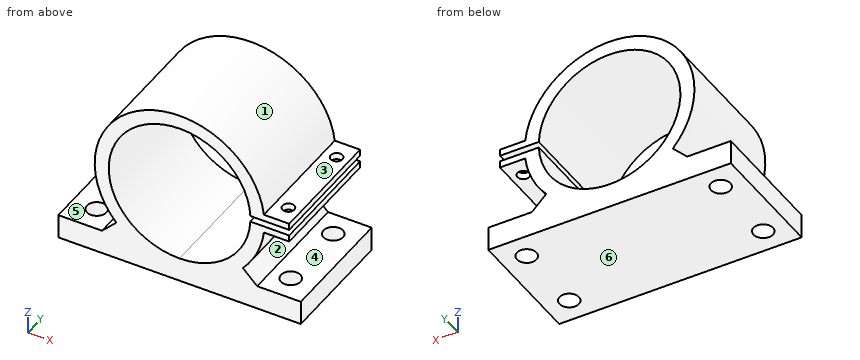
from build123d import *

# Parameters (mm, degrees)
SKETCH1_W           = 3
SKETCH1_H           = 5.08
SKETCH1_W_2         = 1.910737821
SKETCH1_W_3         = 5
SKETCH1_H_2         = 6.35
SKETCH1_W_4         = 3.175
BOSS_EXTRUDE1_DEPTH = 31.75
SKETCH2_W           = 21.412406597
SKETCH2_H           = 1.5875
CUT_EXTRUDE1_DEPTH  = 31.75
CUT_EXTRUDE2_REACH  = 54.622
SKETCH3_R           = 1.55
SKETCH4_R           = 2.55
CUT_EXTRUDE3_DEPTH  = 31.75


with BuildPart() as part:
    # Sketch1 → Boss-Extrude1 (new body)
    with BuildSketch(Plane(origin=(0, 0, 0), x_dir=(1, 0, 0), z_dir=(0, 1, 0))):
        with BuildLine():
            ThreePointArc((18.55, 0), (-13.116830791, -13.116830791), (0, 18.55))
            Line((0, 18.55), (-12.241246873, 18.55))
            ThreePointArc((-12.241246873, 18.55), (-14.529510105, 16.817965427), (-16.575509472, 14.805509472))
            ThreePointArc((-16.575509472, 14.805509472), (-9.098891287, -20.277100442), (22.079380086, -2.54))
            Line((22.079380086, -2.54), (18.55, -2.54))
            Line((18.55, -2.54), (18.55, 0))
        make_face()
        with BuildLine():
            Line((12.241246873, 18.55), (0, 18.55))
            ThreePointArc((0, 18.55), (13.116830791, 13.116830791), (18.55, 0))
            Line((18.55, 0), (18.55, 2.54))
            Line((18.55, 2.54), (22.079380086, 2.54))
            ThreePointArc((22.079380086, 2.54), (20.277100442, 9.098891287), (16.575509472, 14.805509472))
            ThreePointArc((16.575509472, 14.805509472), (14.529510105, 16.817965427), (12.241246873, 18.55))
        make_face()
        with BuildLine():
            Line((18.55, 2.54), (18.55, 0))
            Line((18.55, 0), (18.55, -2.54))
            Line((18.55, -2.54), (22.079380086, -2.54))
            ThreePointArc((22.079380086, -2.54), (22.188565157, -1.27208541), (22.225, 0))
            ThreePointArc((22.225, 0), (22.188565157, 1.27208541), (22.079380086, 2.54))
            Line((22.079380086, 2.54), (18.55, 2.54))
        make_face()
        with BuildLine():
            ThreePointArc((22.225, 0), (22.188565157, -1.27208541), (22.079380086, -2.54))
            Line((22.079380086, -2.54), (23.799262179, -2.54))
            Line((23.799262179, -2.54), (23.799262179, 2.54))
            Line((23.799262179, 2.54), (22.079380086, 2.54))
            ThreePointArc((22.079380086, 2.54), (22.188565157, 1.27208541), (22.225, 0))
        make_face()
        with Locations((25.299262179, 0)):
            Rectangle(SKETCH1_W, SKETCH1_H)
        with Locations((27.75463109, 0)):
            Rectangle(SKETCH1_W_2, SKETCH1_H)
        with BuildLine():
            Line((-20.32, 18.55), (-12.241246873, 18.55))
            ThreePointArc((-12.241246873, 18.55), (0, 22.225), (12.241246873, 18.55))
            Line((12.241246873, 18.55), (20.32, 18.55))
            Line((20.32, 18.55), (31.75, 18.55))
            Line((31.75, 18.55), (31.75, 24.9))
            Line((31.75, 24.9), (-23.575, 24.9))
            Line((-23.575, 24.9), (-23.575, 18.55))
            Line((-23.575, 18.55), (-20.32, 18.55))
        make_face()
        with BuildLine():
            Line((-12.241246873, 18.55), (0, 18.55))
            Line((0, 18.55), (12.241246873, 18.55))
            ThreePointArc((12.241246873, 18.55), (0, 22.225), (-12.241246873, 18.55))
        make_face()
        with BuildLine():
            Line((20.32, 18.55), (12.241246873, 18.55))
            ThreePointArc((12.241246873, 18.55), (14.529510105, 16.817965427), (16.575509472, 14.805509472))
            Line((16.575509472, 14.805509472), (20.32, 18.55))
        make_face()
        with BuildLine():
            ThreePointArc((-16.575509472, 14.805509472), (-14.529510105, 16.817965427), (-12.241246873, 18.55))
            Line((-12.241246873, 18.55), (-20.32, 18.55))
            Line((-20.32, 18.55), (-16.575509472, 14.805509472))
        make_face()
        with Locations((-26.075, 21.725)):
            Rectangle(SKETCH1_W_3, SKETCH1_H_2)
        with Locations((-30.1625, 21.725)):
            Rectangle(SKETCH1_W_4, SKETCH1_H_2)
    extrude(amount=BOSS_EXTRUDE1_DEPTH)

    # Sketch2 → Cut-Extrude1 (cut)
    with BuildSketch(Plane(origin=(0, 31.75, 0), x_dir=(1, 0, 0), z_dir=(0, 1, 0))):
        with Locations((22.027012195, 0)):
            Rectangle(SKETCH2_W, SKETCH2_H)
    extrude(amount=-CUT_EXTRUDE1_DEPTH, mode=Mode.SUBTRACT)

    # Cut-Extrude2: up to this face of the body (flat: up to its plane)
    cut_extrude2_end = Plane(part.part.faces().sort_by_distance((25.394690043, 15.875, -2.54))[0])
    # Sketch3 → Cut-Extrude2 (cut, up to the picked face)
    with BuildSketch(Plane.XY.offset(2.54), mode=Mode.PRIVATE) as cut_extrude2_sk1:
        with Locations((25.535, 5.08)):
            Circle(SKETCH3_R)
    cut_extrude2_tool1 = split(extrude(cut_extrude2_sk1.sketch, amount=-CUT_EXTRUDE2_REACH, mode=Mode.PRIVATE), bisect_by=cut_extrude2_end, keep=Keep.BOTH, mode=Mode.PRIVATE)
    # Sketch3 → Cut-Extrude2 (cut, up to the picked face)
    with BuildSketch(Plane.XY.offset(2.54), mode=Mode.PRIVATE) as cut_extrude2_sk2:
        with Locations((25.535, 26.67)):
            Circle(SKETCH3_R)
    cut_extrude2_tool2 = split(extrude(cut_extrude2_sk2.sketch, amount=-CUT_EXTRUDE2_REACH, mode=Mode.PRIVATE), bisect_by=cut_extrude2_end, keep=Keep.BOTH, mode=Mode.PRIVATE)
    add(cut_extrude2_tool1.solids().sort_by(Axis((25.535, 5.08, 2.54), (0, 0, -1)))[0], mode=Mode.SUBTRACT)
    add(cut_extrude2_tool2.solids().sort_by(Axis((25.535, 26.67, 2.54), (0, 0, -1)))[0], mode=Mode.SUBTRACT)

    # Sketch4 → Cut-Extrude3 (cut)
    with BuildSketch(Plane.XY.offset(-18.55)):
        with Locations((-25.4, 6.35)):
            Circle(SKETCH4_R)
        with Locations((-25.4, 25.4)):
            Circle(SKETCH4_R)
        with Locations((25.4, 25.4)):
            Circle(SKETCH4_R)
        with Locations((25.4, 6.35)):
            Circle(SKETCH4_R)
    extrude(amount=-CUT_EXTRUDE3_DEPTH, mode=Mode.SUBTRACT)


solid = part.part
Build history of the part. All positions in model axes, mm. Face numbers are marked on the shaded views. A direction names the side the tool comes from. Round coordinates to 2 decimals unless told otherwise and drop trailing zeros. Loops run counter-clockwise (first coordinate to the right, second up) from the corner with the lowest first, then second, coordinate; pieces in that order, holes last. Notation, with made-up numbers: (33.25, -31.75) -> (54.25, -31.75) arc R13 ccw to (54.25, -24.75) -> close; hole circle Ø4 at (-38, -7). An arc over 180 degrees is marked (long way). One line per item, written item: value. Start each with the question number.
Q1. Drop flat-ended pins along their axis: pin 1 Ø6 at (y, z) = (13.5, -9) entering from -X; pin 2 Ø5 at (x, y) = (-20.5, 25.5) entering from +Z; pin 3 Ø1.4 at (y, z) = (8, 1.5) entering from +X. Give the stop position or say it passes through.
Q2. Cut at B-B on z = -6.5. List the corners of the cut face in (x, y), plus the area to 3 significant figures.
Q3. Probe line 1 along Z through (x, y) = (26.5, 10.5); line 2 along Y through (x, z) = (-25.4, -20.25); line 3 along X through (y, z) = (24, -20). List the from-to ranges inside material, lowest first.
Q4. Two-plate mould, pull along Z, no slides. Class the marked faces 3, 4, 5 and 6: released by +Z, released by -Z, zero draft, split by the parting line, or undercut.
Q5. 3-axis set-ups, long thin cutter, end or side, ignore diameter. For the marked faces 1 and 2: which of +Z, -Z, +X, -X, +Y, -Y reach the whole face in a straight line?
Q6. Cut at A-A on x = -25.4. List the corners of the cut face in (y, z), plus the area to 3 significant figures.
Q7. Cut at C-C on y = 5.08. Count the separate pieces of the cut face and the enclosed holes in it, plus the area to 3 significant figures.
Computed:
1. pin 1: x = -21.4
1. pin 2: z = 13.04
1. pin 3: x = 28.71
2. outline: (-21.25, 0) -> (-17.37, 0) -> (-17.37, 31.75) -> (-21.25, 31.75) -> close; (17.37, 0) -> (21.25, 0) -> (21.25, 31.75) -> (17.37, 31.75) -> close
2. area: 246 mm²
3. line 1: -24.9 to -18.55, -2.54 to -0.79, 0.79 to 2.54
3. line 2: 0 to 3.8, 8.9 to 22.85, 27.95 to 31.75
3. line 3: -31.75 to -27.53, -23.27 to 23.27, 27.53 to 31.75
4. face 3: released by +Z
4. face 4: undercut
4. face 5: undercut
4. face 6: released by -Z
5. face 1: +Y, -Y
5. face 2: +X, +Y, -Y
6. outline: (0, -24.9) -> (3.8, -24.9) -> (3.8, -18.55) -> (0, -18.55) -> close; (8.9, -24.9) -> (22.85, -24.9) -> (22.85, -18.55) -> (8.9, -18.55) -> close; (27.95, -24.9) -> (31.75, -24.9) -> (31.75, -18.55) -> (27.95, -18.55) -> close
6. area: 137 mm²
7. separate pieces: 5
7. enclosed holes: 0
7. area: 792 mm²
